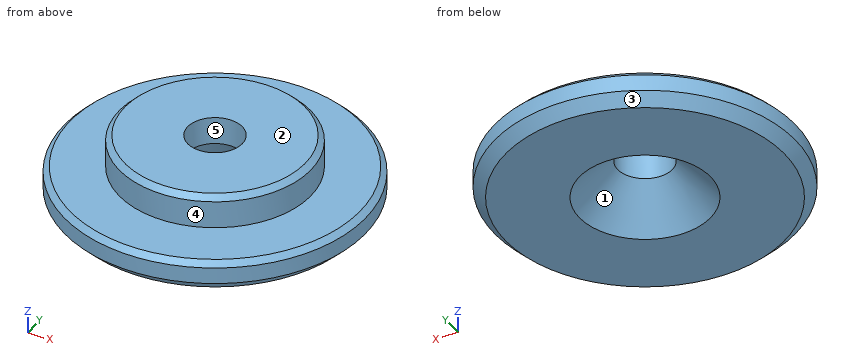
```python
from build123d import *

# Parameters (mm, degrees)
CHAFL_N1_SIZE = 2
CHAFL_N2_SIZE = 1


with BuildPart() as part:
    # Croquis1 → Revolución1 (revolve)
    with BuildSketch(Plane(origin=(0, 0, 0), x_dir=(1, 0, 0), z_dir=(0, 1, 0))):
        Polygon((17.512143261, -5.969981855), (27.512147725, -5.969981855), (27.512147725, 0.030018145), (12.012147715, 0.030018145), (5.012147715, -6.969981855), (5.012147715, -11.969981855), (17.512143261, -11.969981855), align=None)
    revolve(axis=Axis((0.012147715, 0, 0), (0, 0, 1)))

    # Chaflán1
    chafl_n1_edges = [part.edges().sort_by_distance(p)[0] for p in [
        (-27.487852294, 0, -0.030018145),
    ]]
    chamfer(chafl_n1_edges, length=CHAFL_N1_SIZE)

    # Chaflán2
    chafl_n2_edges = [part.edges().sort_by_distance(p)[0] for p in [
        (-27.487852294, 0, 5.969981855),
        (-17.48784783, 0, 11.969981855),
    ]]
    chamfer(chafl_n2_edges, length=CHAFL_N2_SIZE)


solid = part.part
```
Here's how the part is built. I have some questions about the finished solid (model axes, mm). Face numbers are marked on the shaded views. A direction names the side the tool comes from. Coordinates: 2 decimals unless noted, no trailing zeros. Write each loop counter-clockwise with the first axis right and the second up, starting at its lowest first coordinate (ties: lowest second). Pieces come first, ordered by that corner, then holes. Notation, with made-up numbers: (53, 38.5) - (83, 38.5) arc R18 ccw to (83, 62.5) - close; hole circle Ø1 at (79, 42.5). An arc over 180 degrees is marked (long way). One line per item, written item: value.
1) We'd pull the mould along Y, two halves only. Please class the marked faces 1, 2 and 3: pulls with the +Y half, pulls with the -Y half, needs draft (parallel to the pull), parting line crosses it, or undercut.
Model answer:
face 1: undercut
face 2: needs draft
face 3: parting line crosses it
2) On a 3-axis mill with a long thin cutter (end or side, diameter ignored), from which of +Z, -Z, +X, -X, +Y, -Y can I reach the whole of each face in a straight line? I mean the marked faces 4 and 5. Say none if no direction works.
Model answer:
face 4: +Z
face 5: +Z, -Z
3) I need wall thicknesses on line 1 along Z through (x, y) = (15.5, -20); line 2 along Y through (x, z) = (0.5, 9); line 3 along X through (y, z) = (-2, 10.25). Which ranges of each line are inside material? Lowest first, please.
Model answer:
line 1: z = -0.03 to 5.97
line 2: y = -17.49 to -4.98, 4.98 to 17.49
line 3: x = -17.37 to -4.57, 4.59 to 17.4
4) I'm going to push flat-ended pins straight in: P1, Ø6, axis at x = 13.5, z = 5, coming from the +Y side; P2, Ø4, axis at x = -2.5, y = -8, coming from the -Z side; P3, Ø4, axis at y = -15, z = 2.5, coming from the +X side; P4, Ø9, axis at x = 0.01, y = 0, coming from the -Z side. Where does each tip first touch, or does it pass through?
Model answer:
P1: stops at y = 25.42
P2: stops at z = 1.58
P3: stops at x = 24.25
P4: passes through
5) Suppose I cut it at A-A on y = 0. Write out the boundary of the cut face in (x, z).
Model answer:
outline: (-27.49, 1.97) - (-25.49, -0.03) - (-11.99, -0.03) - (-4.99, 6.97) - (-4.99, 11.97) - (-16.49, 11.97) - (-17.49, 10.97) - (-17.49, 5.97) - (-26.49, 5.97) - (-27.49, 4.97) - close; (5.01, 6.97) - (12.01, -0.03) - (25.51, -0.03) - (27.51, 1.97) - (27.51, 4.97) - (26.51, 5.97) - (17.51, 5.97) - (17.51, 10.97) - (16.51, 11.97) - (5.01, 11.97) - close
6) Suppose I cut it at B-B on z = 1. Write out the boundary of the cut face in (x, y).
Model answer:
outline: circle Ø53.06 at (0.01, 0); hole circle Ø21.94 at (0.01, 0)
